Could you check a few things on this model? Use its own coordinates, in mm. Face numbers are marked on the shaded views. A direction names the side the tool comes from. Round coordinates to 2 decimals unless told otherwise and drop trailing zeros. Write each loop counter-clockwise with the first axis right and the second up, starting at its lowest first coordinate (ties: lowest second). Pieces come first, ordered by that corner, then holes. Notation, with made-up numbers: (-18, -1) -> (21, -1) arc R8 ccw to (21, 7) -> close; hole circle Ø10 at (27, 48.25). An arc over 180 degrees is marked (long way). One line per question, with ' | ' between items. Start each with the question number.
1. Imagine slicing it at B-B, the plane y = 55. List the corners of the cut face in (x, z) for me, and give its area (3 significant figures).
2. For the marked faces 1 and 2, which set-ups out of +Z, -Z, +X, -X, +Y, -Y let a thin tool reach every point of the face, with its end or its side?
3. Thinking about a two-plate mould opening in X: for the marked faces 3, 4 and 5, which applies, released by +X, released by -X, zero draft, split by the parting line, or undercut?
4. For pin 1 Ø3 at (y, z) = (57, -4.5) entering from -X; pin 2 Ø5 at (x, z) = (-25.5, -1.5) entering from -Y, each with a flat end and sliding along its axis, tell me the tip position at first contact or that it passes through.
5. Imagine slicing it at D-D, the plane x = 2. List the corners of the cut face in (y, z) for me.
6. If I drill on line 1 along Y through (x, z) = (-20, -4.25); line 2 along X through (y, z) = (52.5, -2.25); line 3 along X through (y, z) = (50, -5), over which ranges is the centre line in solid material (lowest first)? Write a range as [from, to].
7. Imagine slicing it at A-A, the plane x = -20. List the corners of the cut face in (y, z) for me, and give its area (3 significant figures).
8. Imagine slicing it at C-C, the plane z = -2.5. List the corners of the cut face in (x, y) for me.
from build123d import *

# Parameters (mm, degrees)
BASE_EXTRUDE_DEPTH = 10
SKETCH2_R          = 5
CUT_EXTRUDE1_DEPTH = 11
FILLET1_R          = 5


with BuildPart() as part:
    # Sketch1 → Base-Extrude (new body)
    with BuildSketch(Plane.XY):
        with BuildLine():
            Line((17.145241183, 27.717792456), (28.25998861, 44.344950651))
            Line((28.25998861, 44.344950651), (-14.878235452, 64.026276153))
            ThreePointArc((-14.878235452, 64.026276153), (-30.761612778, 60.763930789), (-32.493423944, 44.641728625))
            Line((-32.493423944, 44.641728625), (-25.781727065, 33.016728625))
            Line((-25.781727065, 33.016728625), (4.666426174, 33.016728625))
            ThreePointArc((4.666426174, 33.016728625), (9.022139107, 32.370395921), (13.002486744, 30.487097271))
            Line((13.002486744, 30.487097271), (17.145241183, 27.717792456))
        make_face()
    extrude(amount=-BASE_EXTRUDE_DEPTH)

    # Sketch2 → Cut-Extrude1 (cut, through all)
    with BuildSketch(Plane(origin=(0, 0, -10), x_dir=(-1, 0, 0), z_dir=(0, 0, -1))):
        with Locations((20.585574642, 51.516728625)):
            Circle(SKETCH2_R)
    extrude(amount=-CUT_EXTRUDE1_DEPTH, mode=Mode.SUBTRACT)

    # Fillet1
    fillet1_edges = [part.edges().sort_by_distance(p)[0] for p in [
        (28.25998861, 44.344950651, -5),
    ]]
    fillet(fillet1_edges, radius=FILLET1_R)


solid = part.part
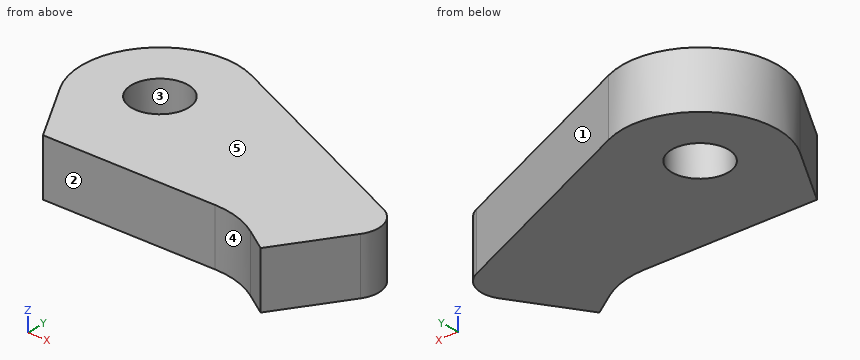
Geometry results:
1) outline: (-33.89, -10) -> (-24.17, -10) -> (-24.17, 0) -> (-33.89, 0) -> close; (-17, -10) -> (4.91, -10) -> (4.91, 0) -> (-17, 0) -> close | area: 316 mm2
2) face 1: +Z, -Z, +X, +Y | face 2: +Z, -Z, -X, -Y
3) face 3: undercut | face 4: released by -X | face 5: zero draft
4) pin 1: stops at x = -33.75 | pin 2: stops at y = 33.02
5) outline: (33.02, -10) -> (56.33, -10) -> (56.33, 0) -> (33.02, 0) -> close
6) line 1: y = [33.02, 46.55], [56.48, 65.25] | line 2: x = [-34.3, -25.49], [-15.68, 10.39] | line 3: x = [-34.25, -25.35], [-15.82, 15.87]
7) outline: (33.02, -10) -> (46.55, -10) -> (46.55, 0) -> (33.02, 0) -> close; (56.48, -10) -> (65.25, -10) -> (65.25, 0) -> (56.48, 0) -> close | area: 223 mm2
8) outline: (-32.49, 44.64) -> (-25.78, 33.02) -> (4.67, 33.02) arc R15 cw to (13, 30.49) -> (17.15, 27.72) -> (24.99, 39.46) arc R5 ccw to (22.91, 46.79) -> (-14.88, 64.03) arc R13.75 ccw to start; hole circle Ø10 at (-20.59, 51.52)
